```python
from build123d import *

# Parameters (mm, degrees)
F0_W     = 45
F0_H     = 11.742345
F1_DEPTH = 3
F2_R     = 6
F3_DEPTH = 11.742345
F4_R     = 5


with BuildPart() as f1:
    # F0 (on Top) → F1 (new body)
    with BuildSketch(Plane.XY):
        with Locations((-22.5, 5.8711725)):
            Rectangle(F0_W, F0_H)
    extrude(amount=F1_DEPTH)

    # F2 (on Front) → F3 (join)
    with BuildSketch(Plane.XZ):
        with BuildLine():
            Line((-45, 3), (0, 3))
            Line((0, 3), (-12.3530250157, 7.6497290392))
            ThreePointArc((-12.3530250157, 7.6497290392), (-20, 18), (-27.6469749843, 7.6497290392))
            Line((-27.6469749843, 7.6497290392), (-45, 3))
        make_face()
        with Locations((-20, 10)):
            Circle(F2_R, mode=Mode.SUBTRACT)
    extrude(amount=-F3_DEPTH)

    # F4
    f4_edges = [f1.edges().sort_by_distance(p)[0] for p in [
        (-45, 0, 1.5),
        (0, 0, 1.5),
        (0, 11.742345, 1.5),
        (-45, 11.742345, 1.5),
    ]]
    fillet(f4_edges, radius=F4_R)


solid = f1.part
```
The model under review builds one solid part; all positions refer to its coordinate system, in mm. Round coordinates to 2 decimals unless told otherwise and drop trailing zeros. Write each loop counter-clockwise with the first axis right and the second up, starting at its lowest first coordinate (ties: lowest second). Pieces come first, ordered by that corner, then holes. Notation, with made-up numbers: M 22.25,3.25 L 27.25,3.25 A15 ccw 27.25,8.25 Z; hole C 47,-26.5 d5. An arc over 180 degrees is marked long. Use CSV: the item, a comma, the result in double quotes. Start each with the question number.
(1) For line 1 along Z through (x, y) = (-20, 8.25); line 2 along Z through (x, y) = (-14.5, 0.75); line 3 along X through (y, z) = (11.25, 13), list the stretches that pass through material, from the lowest coordinate up.
(2) We need section D-D, the plane x = -3. State the section outline as (y, z) points.
(3) We need section A-A, the plane x = -20. State the section outline as (y, z) points, then the cut area to 3 significant figures.
(4) We need section C-C, the plane y = 8.75. State the section outline as (x, z) points.
(5) The part is to be moulded in two halves that separate along Z. For faces 1 (the face through (-23, 11.742, 3)), 2 (the face through (-23, 6, 0)), 3 (the face through (-24.76, 5.79, 6.35)), 4 (the face through (-20, 6, 18)), say which applies: +Z half, -Z half, draft (parallel to the pull), parting line (faces both ways), or undercut.
(6) Clearance check with flat-ended pins moving along their axes: P1, Ø3, axis at y = 9, z = 10, coming from the +X side; P2, Ø9.5, axis at x = -20, z = 10, coming from the -Y side; P3, Ø5, axis at y = 6.5, z = 11, coming from the -X side; P4, Ø6, axis at y = 9.5, z = 5, coming from the -X side. State where each tip first meets the part, or that it passes through.
(7) We need section B-B, the plane z = 10. State the section outline as (x, y) points.
Findings:
1,line 1,"0 to 4, 16 to 18"
1,line 2,"0 to 7.6, 12.4 to 15.81"
1,line 3,"-27.42 to -25.2, -14.8 to -12.58"
2,outline,"M 0.42,0 L 11.32,0 L 11.32,4.13 L 0.42,4.13 Z"
3,outline,"M 0,0 L 11.74,0 L 11.74,4 L 0,4 Z; M 0,16 L 11.74,16 L 11.74,18 L 0,18 Z"
3,area,"70.5 mm^2"
4,outline,"M -44.58,0 L -0.42,0 L -0.42,3.16 L -12.35,7.65 A8 ccw long -27.65,7.65 L -44.58,3.11 Z; hole C -20,10 d12"
5,face 1,"draft"
5,face 2,"-Z half"
5,face 3,"undercut"
5,face 4,"undercut"
6,P1,"x = -12"
6,P2,"through"
6,P3,"x = -28"
6,P4,"x = -44.97"
7,outline,"M -28,0 L -26,0 L -26,11.74 L -28,11.74 Z; M -14,0 L -12,0 L -12,11.74 L -14,11.74 Z"
